Autodesk Inventor part; units mm, degrees
ref_plane "YZ Plane" through (0, 0, 0) normal (1, 0, 0) x (0, 1, 0)
ref_plane "XZ Plane" through (0, 0, 0) normal (0, 1, 0) x (-1, 0, 0)
ref_plane "XY Plane" through (0, 0, 0) normal (0, 0, 1) x (1, 0, 0)
sketch "Sketch1" plane through (0, 0, 0) normal (0, 0, 1) x (1, 0, 0)
  line L0 (-13.97, 10.16) -> (0, 10.16)
  line L1 (0, 10.16) -> (0, 0)
  line L2 (0, 0) -> (-13.97, 0)
  line L3 (-13.97, 0) -> (-13.97, 10.16)
  dimension "d0" = 13.97
  dimension "d1" = 10.16
extrude "Extrusion1" add sketch "Sketch1" along normal blind 30.48
sketch "Sketch2" plane through (0, 0, 0) normal (0, 0, -1) x (-1, 0, 0)
  line L0 (13.97, 10.16) -> (0, 10.16)
  line L1 (0, 10.16) -> (0, 0)
  line L2 (0, 0) -> (13.97, 0)
  line L3 (13.97, 0) -> (13.97, 10.16)
  circle A0 centre (2.8956, 5.08) radius 2.8194
  circle A1 centre (11.0744, 5.08) radius 2.8194
  dimension "d4" = 5.6388
  dimension "d5" = 5.6388
  dimension "d6" = 2.54
  dimension "d7" = 5.08
  dimension "d8" = 2.8956
  dimension "d9" = 2.8956
extrude "Extrusion2" cut sketch "Sketch2" against normal blind 27.178 contours A0 | A1
sketch "Sketch3" plane through (0, 0, 0) normal (0, 0, -1) x (-1, 0, 0)
  circle A0 centre (2.8956, 5.08) radius 2.8194
  circle A1 centre (11.0744, 5.08) radius 2.8194
  circle A2 centre (2.8956, 5.08) radius 2.4447
  circle A3 centre (11.0744, 5.08) radius 2.4447
  point P0 (0, 0)
  dimension "d12" = 4.8895
  dimension "d13" = 4.8895
extrude "Extrusion3" cut sketch "Sketch3" against normal blind 33.02 contours A2 | A3
chamfer "Chamfer1" distance 0.2032 angle 45 2 edges at (-0.4509, 5.08, 27.178) (-8.6297, 5.08, 27.178)
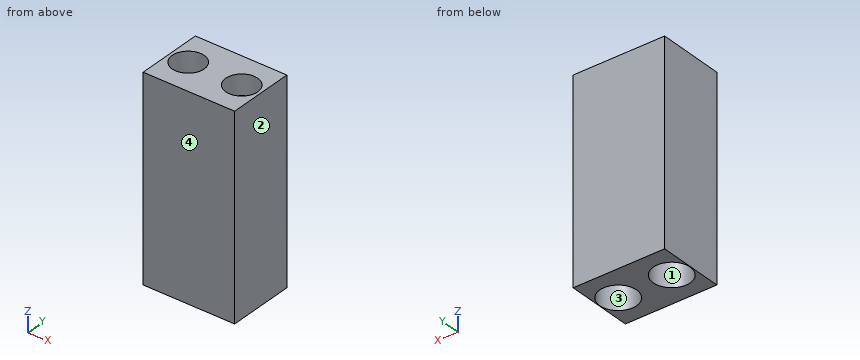
Part model, mm, in its own coordinate system. Face numbers are marked on the shaded views. Round coordinates to 2 decimals unless told otherwise and drop trailing zeros. Write each loop counter-clockwise with the first axis right and the second up, starting at its lowest first coordinate (ties: lowest second). Pieces come first, ordered by that corner, then holes. Notation, with made-up numbers: (-25, 43.5) -> (22, 43.5) arc R24 ccw to (22, 55.5) -> close; hole circle Ø6 at (78.25, -5.5). An arc over 180 degrees is marked (long way). Return JSON: item names as keys, results as strings. Group by question number.
Q1. Pin check, flat tips, straight feed: pin 1 (1.5 mm diameter, centred on x = -6, z = 6, fed in from -Y); pin 2 (5 mm diameter, centred on x = -11.07, y = 5.08, fed in from -Z); pin 3 (1.7 mm diameter, centred on x = -10.5, y = 5.5, fed in from -Z). Stop position of each tip, or through.
Q2. Probe L1, parallel to Y at x = -11, z = 28; L2, parallel to X at y = 7.5, z = 25.5; L3, parallel to X at y = 6.75, z = 23.5. List the from-to ranges inside material, lowest first. Write a range as [from, to].
Q3. Saw through at B-B on z = 18.5. Write the cut outline in (x, y) (3 decimals), plus the area to 3 significant figures.
Q4. Mould opens along X. For the marked faces 1, 2, 3 and 4 say: pulls with the +X half, pulls with the -X half, needs draft (parallel to the pull), parting line crosses it, or undercut.
Q5. Saw through at A-A on y = 5.08. State how many separate pieces and enclosed holes the cut face has, plus the area to 3 significant figures.
Answer:
{
 "1": {"pin 1": "y = 0", "pin 2": "z = 27.32", "pin 3": "through"},
 "2": {"L1": "[0, 2.64], [7.52, 10.16]", "L2": "[-13.97, -12.52], [-9.63, -4.34], [-1.45, 0]", "L3": "[-13.97, -13.35], [-8.8, -5.17], [-0.62, 0]"},
 "3": {"outline": "(-13.97, 0) -> (0, 0) -> (0, 10.16) -> (-13.97, 10.16) -> close; hole circle Ø5.639 at (-11.074, 5.08); hole circle Ø5.639 at (-2.896, 5.08)", "area": "92.0 mm2"},
 "4": {"face 1": "undercut", "face 2": "pulls with the +X half", "face 3": "undercut", "face 4": "needs draft"},
 "5": {"separate pieces": "3", "enclosed holes": "0", "area": "86.9 mm2"}
}
